from build123d import *

# Parameters (mm, degrees)
SKETCH1_W           = 10
SKETCH1_H           = 4
SKETCH1_W_2         = 4
SKETCH1_H_2         = 6
SKETCH1_W_3         = 6
BOSS_EXTRUDE1_DEPTH = 4


with BuildPart() as part:
    # Sketch1 → Boss-Extrude1 (new body)
    with BuildSketch(Plane(origin=(0, 0, 0), x_dir=(0, 0, -1), z_dir=(1, 0, 0))):
        Polygon((-45.126561272, -21.465862465), (41.462435166, -21.465862465), (41.462435166, 37.538855), (6.497816801, 37.538855), (-45.126561272, 6.437068622), align=None)
        with Locations((21.33035671, 33.233983224)):
            Rectangle(SKETCH1_W, SKETCH1_H, mode=Mode.SUBTRACT)
        with Locations((-40.626561272, 3.062484248)):
            Rectangle(SKETCH1_W_2, SKETCH1_H_2, mode=Mode.SUBTRACT)
        with Locations((-40.626561272, -5.437515752)):
            Rectangle(SKETCH1_W_2, SKETCH1_H, mode=Mode.SUBTRACT)
        with Locations((-26.374737007, -16.111091518)):
            Rectangle(SKETCH1_W, SKETCH1_H, mode=Mode.SUBTRACT)
        with Locations((-12.874826786, -16.142516965)):
            Rectangle(SKETCH1_W_3, SKETCH1_H, mode=Mode.SUBTRACT)
        with Locations((34.83035671, 33.233983224)):
            Rectangle(SKETCH1_W_3, SKETCH1_H, mode=Mode.SUBTRACT)
        with Locations((8.963743124, 30.24228943)):
            Rectangle(SKETCH1_W_2, SKETCH1_H_2, mode=Mode.SUBTRACT)
        with Locations((8.963743124, 21.74228943)):
            Rectangle(SKETCH1_W_2, SKETCH1_H, mode=Mode.SUBTRACT)
        with BuildLine():
            Line((-36.652183199, -6.33954665), (-36.652183199, 9.188170503))
            ThreePointArc((-36.652183199, 9.188170503), (-27.502183199, 13.424311927), (-18.352183199, 9.188170503))
            Line((-18.352183199, 9.188170503), (-18.352183199, -6.33954665))
            ThreePointArc((-18.352183199, -6.33954665), (-27.502183199, -10.575688073), (-36.652183199, -6.33954665))
        make_face(mode=Mode.SUBTRACT)
    extrude(amount=BOSS_EXTRUDE1_DEPTH)


solid = part.part
For this review, take the finished solid that the model builds, in its own axes (mm). Give positions to 0.01 mm unless a question says otherwise; leave off trailing zeros. Order: outer loops, then holes, each group sorted by start corner. A loop starts at its lowest first (then second) coordinate and runs counter-clockwise, first axis right, second up. Notation, with made-up numbers: (0, 34) - (6, 34) arc R26 ccw to (6, 56) - close; hole circle Ø11 at (-27, -16). An arc over 180 degrees is marked (long way). Answer as a JSON object with one key per item and string values. Group by question number.
Item 1: Take a section at B-B on y = 3.5. Give the boundary of the cut face in (x, z).
Item 2: Take a section at D-D on z = 23. Give the boundary of the cut face in (x, y).
Item 3: Take a section at C-C on x = 3.15. Give the number of separate pieces and of enclosed holes in the cut face, and give its area (3 significant figures).
Item 4: Wall thickness on line 1 along Z through (x, y) = (2.75, 5); line 2 along Y through (x, z) = (0.5, -9.5); line 3 along Y through (x, z) = (3.6, -24.5): over which ranges is each line inside the solid? List them lowest first.
Item 5: Take a section at A-A on z = -21. Give the boundary of the cut face in (x, y).
Item 6: Draft analysis for pull direction Z (two halves, no side actions). For faces 1 (the flat face through (0, 2, -7)), 2 (the flat face through (2, -3.438, 41)), state which applies: pulls with the +Z half, pulls with the -Z half, needs draft (parallel to the pull), parting line crosses it, or undercut.
Reported:
{
 "1": {"outline": "(0, -41.46) - (4, -41.46) - (4, 18.35) - (0, 18.35) - close; (0, 36.65) - (4, 36.65) - (4, 38.63) - (0, 38.63) - close; (0, 42.63) - (4, 42.63) - (4, 45.13) - (0, 45.13) - close"},
 "2": {"outline": "(0, -21.47) - (4, -21.47) - (4, -18.11) - (0, -18.11) - close; (0, -14.11) - (4, -14.11) - (4, -9.7) - (0, -9.7) - close; (0, 12.55) - (4, 12.55) - (4, 19.77) - (0, 19.77) - close"},
 "3": {"separate pieces": "1", "enclosed holes": "9", "area": "3,710 mm^2"},
 "4": {"line 1": "-41.46 to 18.35, 36.65 to 38.63, 42.63 to 45.13", "line 2": "-21.47 to 19.74, 23.74 to 27.24, 33.24 to 37.54", "line 3": "-21.47 to 31.23, 35.23 to 37.54"},
 "5": {"outline": "(0, -21.47) - (4, -21.47) - (4, 31.23) - (0, 31.23) - close; (0, 35.23) - (4, 35.23) - (4, 37.54) - (0, 37.54) - close"},
 "6": {"face 1": "needs draft", "face 2": "undercut"}
}
